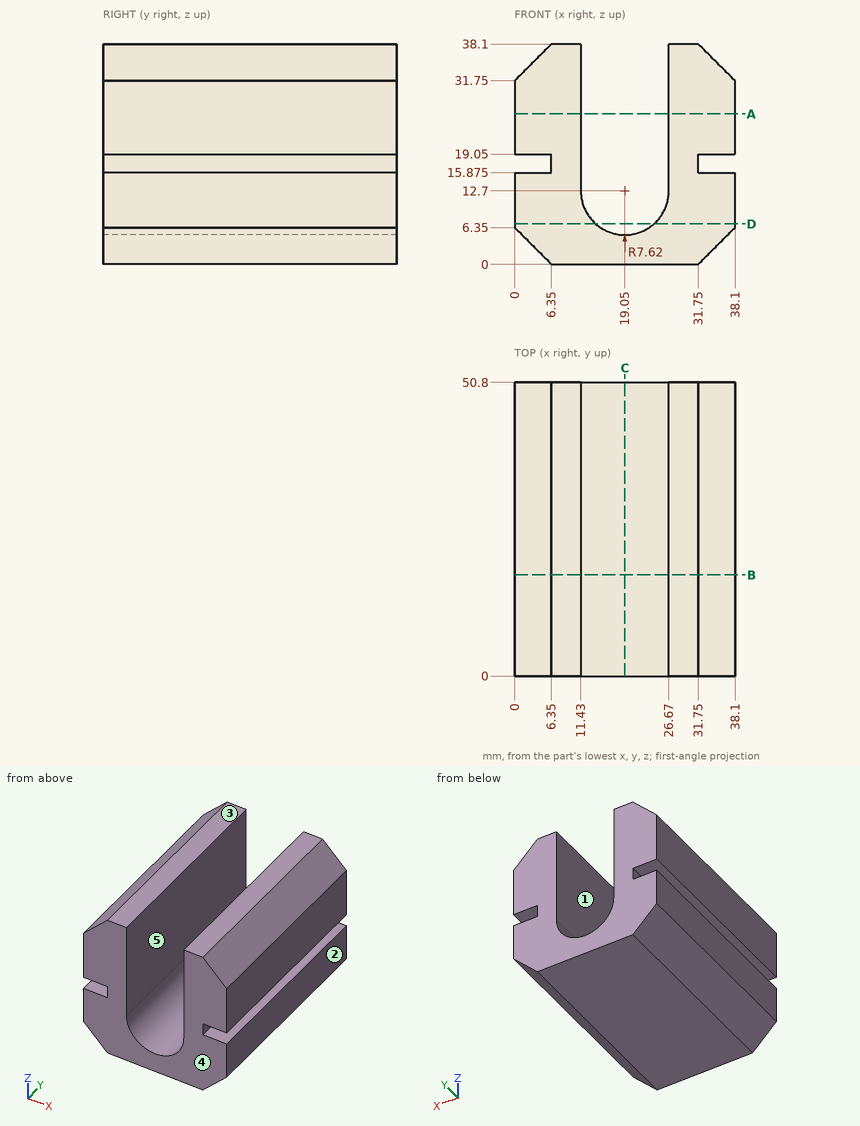
Design review of the part shown in the three views and the two pictorial views. Dimensions are in mm from the part's minimum x, y and z. A direction names the side the tool comes from. Round coordinates to 2 decimals unless told otherwise and drop trailing zeros. Write each loop counter-clockwise with the first axis right and the second up, starting at its lowest first coordinate (ties: lowest second). Pieces come first, ordered by that corner, then holes. Notation, with made-up numbers: (55.5, 1.5) -> (94.5, 1.5) arc R10 cw to (94.5, 14.5) -> close; hole circle Ø10 at (30.25, -25). An arc over 180 degrees is marked (long way). Answer as a JSON object with one key per item and string values.
1. Machinability: for the marked faces 4 and 5, which of the approach directions +Z, -Z, +X, -X, +Y, -Y give a long, thin tool a straight path to every point of the face, cutting with its end or side? Answer none if there is none.
Results found:
{"face 4": "+Z, -Z, +X, -X, -Y", "face 5": "+Z, +Y, -Y"}
2. The part is to be moulded in two halves that separate along X. For the marked faces 1, 2 and 3, say which applies: pulls with the +X half, pulls with the -X half, needs draft (parallel to the pull), parting line crosses it, or undercut.
Results found:
{"face 1": "undercut", "face 2": "pulls with the +X half", "face 3": "needs draft"}
3. Clearance check with flat-ended pins moving along their axes: pin 1 (1 mm diameter, centred on y = 32, z = 17, fed in from -X); pin 2 (3 mm diameter, centred on x = 4, y = 16, fed in from -Z); pin 3 (1 mm diameter, centred on y = 18.5, z = 17, fed in from +X). State where each tip first meets the part, or that it passes through.
Results found:
{"pin 1": "stops at x = 6.35", "pin 2": "stops at z = 0.85", "pin 3": "stops at x = 31.75"}
4. We need section A-A on z = 26. State the section outline as (x, y) points, and give its area (3 significant figures).
Results found:
{"outline": "(0, 0) -> (11.43, 0) -> (11.43, 50.8) -> (0, 50.8) -> close; (26.67, 0) -> (38.1, 0) -> (38.1, 50.8) -> (26.67, 50.8) -> close", "area": "1,160 mm^2"}
5. We need section D-D on z = 7. State the section outline as (x, y) points, and give its area (3 significant figures).
Results found:
{"outline": "(0, 0) -> (13.99, 0) -> (13.99, 50.8) -> (0, 50.8) -> close; (24.11, 0) -> (38.1, 0) -> (38.1, 50.8) -> (24.11, 50.8) -> close", "area": "1,420 mm^2"}
6. We need section C-C on x = 19.05. State the section outline as (y, z) points, and give its area (3 significant figures).
Results found:
{"outline": "(0, 0) -> (50.8, 0) -> (50.8, 5.08) -> (0, 5.08) -> close", "area": "258 mm^2"}
7. To check wall thickness, follow line 1 along X through (y, z) = (23, 18.5); line 2 along X through (y, z) = (39.5, 25); line 3 along Z through (x, y) = (35, 36.5) (3 decimals). State the ranges of each line that lie inside material, in increasing order.
Results found:
{"line 1": "x = 6.35 to 11.43, 26.67 to 31.75", "line 2": "x = 0 to 11.43, 26.67 to 38.1", "line 3": "z = 3.25 to 15.875, 19.05 to 34.85"}
8. We need section B-B on y = 17.5. State the section outline as (x, z) points (3 decimals), and give its area (3 significant figures).
Results found:
{"outline": "(0, 6.35) -> (6.35, 0) -> (31.75, 0) -> (38.1, 6.35) -> (38.1, 15.875) -> (31.75, 15.875) -> (31.75, 19.05) -> (38.1, 19.05) -> (38.1, 31.75) -> (31.75, 38.1) -> (26.67, 38.1) -> (26.67, 12.7) arc R7.62 cw to (11.43, 12.7) -> (11.43, 38.1) -> (6.35, 38.1) -> (0, 31.75) -> (0, 19.05) -> (6.35, 19.05) -> (6.35, 15.875) -> (0, 15.875) -> close", "area": "852 mm^2"}
